Input: part model. Units: mm. Frame: model coordinates. A direction names the side the tool comes from. Give positions to 0.01 mm unless a question says otherwise; leave off trailing zeros. Order: outer loops, then holes, each group sorted by start corner. A loop starts at its lowest first (then second) coordinate and runs counter-clockwise, first axis right, second up. Notation, with made-up numbers: (-11, -15.75) - (30, -15.75) arc R14 ccw to (30, 1.25) - close; hole circle Ø10 at (69.25, 21.5). An arc over 180 degrees is marked (long way). Use a Markdown table: item, result.
Autodesk Inventor part; units mm, degrees
ref_plane "YZ Plane" through (0, 0, 0) normal (1, 0, 0) x (0, 1, 0)
ref_plane "XZ Plane" through (0, 0, 0) normal (0, 1, 0) x (-1, 0, 0)
ref_plane "XY Plane" through (0, 0, 0) normal (0, 0, 1) x (1, 0, 0)
sketch "Sketch1" plane through (0, 0, 0) normal (0, 0, 1) x (1, 0, 0)
  line L0 (-46.8353, 30.48) -> (46.8353, 30.48)
  arc A0 (0, 55.88) -> (-46.8353, 30.48) centre (0, 0) ccw
  arc A1 (46.8353, 30.48) -> (0, 55.88) centre (0, 0) ccw
extrude "Extrusion1" add sketch "Sketch1" against normal blind 12.7
sketch "Sketch2" plane through (0, 0, 0) normal (0, 0, 1) x (1, 0, 0)
  line L0 (-46.8353, 30.48) -> (46.8353, 30.48)
  arc A0 (46.8353, 30.48) -> (-46.8353, 30.48) centre (0, 0) ccw
  line L1 (0, 55.88) -> (0, 0)
  line L2 (0, 0) -> (46.8353, 30.48)
  line L3 (-46.8353, 30.48) -> (0, 0)
  line L4 (0, 0) -> (-26.6416, 49.1203)
  line L5 (0, 0) -> (26.6416, 49.1203)
  line L6 (-16.5866, 48.9387) -> (-20.0564, 52.6491)
  line L7 (-20.0564, 52.6491) -> (-18.578, 57.5092)
  line L8 (-18.578, 57.5092) -> (-13.6298, 58.659)
  line L9 (-13.6298, 58.659) -> (-10.16, 54.9486)
  line L10 (-10.16, 54.9486) -> (-11.6384, 50.0885)
  line L11 (-11.6384, 50.0885) -> (-16.5866, 48.9387)
  line L12 (16.5866, 48.9387) -> (11.6384, 50.0885)
  line L13 (11.6384, 50.0885) -> (10.16, 54.9486)
  line L14 (10.16, 54.9486) -> (13.6298, 58.659)
  line L15 (13.6298, 58.659) -> (18.578, 57.5092)
  line L16 (18.578, 57.5092) -> (20.0564, 52.6491)
  line L17 (20.0564, 52.6491) -> (16.5866, 48.9387)
  line L18 (11.6384, 50.0885) -> (16.5866, 48.9387)
  line L19 (16.5866, 48.9387) -> (16.1555, 47.0836)
  line L20 (16.1555, 47.0836) -> (11.2073, 48.2333)
  line L21 (11.2073, 48.2333) -> (11.6384, 50.0885)
  line L22 (-16.5866, 48.9387) -> (-11.6384, 50.0885)
  line L23 (-11.6384, 50.0885) -> (-11.2072, 48.2329)
  line L24 (-11.2072, 48.2329) -> (-16.1554, 47.0832)
  line L25 (-16.1554, 47.0832) -> (-16.5866, 48.9387)
  line L26 (-17.0874, 49.4743) -> (-11.425, 50.79)
  line L27 (11.425, 50.79) -> (17.0874, 49.4743)
  point P0 (-15.1082, 53.7989)
  point P1 (15.1082, 53.7989)
  dimension "d8" = 28.47
  dimension "d9" = 28.47
  dimension "d18" = 5.08
  dimension "d19" = 5.08
  dimension "d20" = 10.16
  dimension "d21" = 10.16
  dimension "d22" = 1.905
  dimension "d23" = 1.9046
  dimension "d24" = 0.635
  dimension "d25" = 0.635
extrude "Extrusion2" cut sketch "Sketch2" against normal blind 12.7 contours A0 L4 L0 | L0 L4 L3 | L5 L0 L2 | L6 L7 L8 L9 A0 | A0 L10 L26 L6 | L0 L5 A0 | L14 L15 L16 L17 A0 | A0 L17 L27 L13 | L11 L23 L24 L25 | L12 L19 L20 L21
sketch "Sketch3" plane through (-17.0874, 49.4743, 0) normal (-0.2263272, 0.9740513, 0) x (0.9740513, 0.2263272, 0)
  line L0 (0, 0) -> (0, 12.7)
  line L1 (1.0016, 8.763) -> (1.0016, 4.4937)
  line L2 (1.0016, 4.4937) -> (4.8116, 4.4937)
  line L3 (4.8116, 4.4937) -> (4.8116, 8.763)
  line L4 (4.8116, 8.763) -> (1.0016, 8.763)
  point P0 (5.8132, 12.7)
  point P1 (5.4466, 0)
  dimension "d28" = 0.635
  dimension "d29" = 3.81
  dimension "d30" = 3.937
extrude "Extrusion3" cut sketch "Sketch3" against normal up to next
sketch "Sketch4" plane through (11.425, 50.79, 0) normal (0.2263272, 0.9740513, 0) x (0.9740513, -0.2263272, 0)
  line L0 (0, 0) -> (0, 12.7)
  line L1 (0.635, 8.763) -> (0.635, 4.4958)
  line L2 (0.635, 4.4958) -> (4.445, 4.4958)
  line L3 (4.445, 4.4958) -> (4.445, 8.763)
  line L4 (4.445, 8.763) -> (0.635, 8.763)
  point P0 (0.3666, 0)
  dimension "d33" = 3.81
  dimension "d34" = 3.937
  dimension "d35" = 0.635
  dimension "d36" = 4.2672
extrude "Extrusion4" cut sketch "Sketch4" against normal up to next
sketch "Sketch5" plane through (0, 0, -12.7) normal (0, 0, -1) x (-1, 0, 0)
  line L0 (16.5316, 30.48) -> (-16.5316, 30.48)
  line L1 (-16.5316, 30.48) -> (16.5316, 30.48)
  line L2 (16.5316, 30.48) -> (16.5316, 33.655)
  line L3 (16.5316, 33.655) -> (-16.5316, 33.655)
  line L4 (-16.5316, 33.655) -> (-16.5316, 30.48)
  dimension "d39" = 3.175
extrude "Extrusion5" add sketch "Sketch5" along normal blind 9.525
sketch "Sketch7" plane through (-16.5316, 33.655, -12.7) normal (0, 1, 0) x (1, 0, 0)
  line L0 (33.0631, 9.525) -> (0, 9.525)
  line L1 (0, 9.525) -> (33.0631, 9.525)
  line L2 (33.0631, 9.525) -> (33.0631, 6.35)
  line L3 (33.0631, 6.35) -> (0, 6.35)
  line L4 (0, 6.35) -> (0, 9.525)
  point P0 (16.5316, -12.7)
  dimension "d42" = 3.175
extrude "Extrusion6" add sketch "Sketch7" along normal blind 6.35
sketch "Sketch8" plane through (0, 0, 0) normal (0, 0, 1) x (1, 0, 0)
  line L0 (-16.5316, 30.48) -> (16.5316, 30.48)
  line L1 (-16.5316, 30.48) -> (16.5316, 30.48)
  line L2 (16.5316, 30.48) -> (16.5316, 33.655)
  line L3 (16.5316, 33.655) -> (-16.5316, 33.655)
  line L4 (-16.5316, 33.655) -> (-16.5316, 30.48)
  dimension "d45" = 3.175
extrude "Extrusion7" add sketch "Sketch8" along normal blind 9.525
sketch "Sketch9" plane through (-16.5316, 33.655, 0) normal (0, 1, 0) x (1, 0, 0)
  line L0 (0, -9.525) -> (33.0631, -9.525)
  line L1 (0, -9.525) -> (33.0631, -9.525)
  line L2 (33.0631, -9.525) -> (33.0631, -6.35)
  line L3 (33.0631, -6.35) -> (0, -6.35)
  line L4 (0, -6.35) -> (0, -9.525)
  point P0 (16.5316, 0)
  dimension "d48" = 3.175
extrude "Extrusion8" add sketch "Sketch9" along normal blind 6.35
properties part number "IR Sensor Piece Ver 2"
1. Mould query, pull axis X, two halves, no side actions, for faces 6 (the face through (11.42, 49.15, -6.26)), 7 (the face through (-23.185, 50.843, -6.261)), 8 (the face through (16.374, 48.024, -6.261)), 9 (the face through (23.28, 50.8, -6.26)). Classes: pulls with the +X half, pulls with the -X half, needs draft (parallel to the pull), parting line crosses it, or undercut.
Response:
| item | result |
|---|---|
| face 6 | undercut |
| face 7 | pulls with the -X half |
| face 8 | undercut |
| face 9 | pulls with the +X half |
2. Material intervals for line 1 along Z through (x, y) = (-6, 36.25) (3 decimals); line 2 along Z through (x, y) = (-15.5, 40.25); line 3 along Y through (x, z) = (13.5, -20) (3 decimals), sorted ascending.
Response:
| item | result |
|---|---|
| line 1 | z = -22.225 to -19.05, -12.7 to 0, 6.35 to 9.525 |
| line 2 | z = -12.7 to 0 |
| line 3 | y = 30.48 to 40.005 |
3. Section query A-A (y = 38.75). State how many separate pieces and enclosed holes the cut face has, then the cut area to 3 significant figures.
Response:
| item | result |
|---|---|
| separate pieces | 3 |
| enclosed holes | 0 |
| area | 744 mm^2 |
4. Pin query (flat end, axial travel): pin 1 (3 mm diameter, centred on x = -7, z = 4.5, fed in from +Y) (3 decimals); pin 2 (3 mm diameter, centred on x = 9.5, z = -10.5, fed in from +Y); pin 3 (0.7 mm diameter, centred on x = 14, y = 49.5, fed in from +Z). Return the tip coordinate at first contact, or that it passes through.
Response:
| item | result |
|---|---|
| pin 1 | stops at y = 33.655 |
| pin 2 | stops at y = 55.3 |
| pin 3 | stops at z = 0 |
5. Section query B-B (x = -4). Return loops of the section in (y, z) (3 decimals).
Response:
| item | result |
|---|---|
| outline | (30.48, -22.225) - (40.005, -22.225) - (40.005, -19.05) - (33.655, -19.05) - (33.655, -12.7) - (55.737, -12.7) - (55.737, 0) - (33.655, 0) - (33.655, 6.35) - (40.005, 6.35) - (40.005, 9.525) - (30.48, 9.525) - close |
6. Set-up query: faces 1 (the face through (0, 40.005, -21)), 2 (the face through (15.8, 49.12, -6.26)), 3 (the face through (16.104, 49.703, -6.261)), 4 (the face through (-16.532, 34, 7)), 5 (the face through (0, 33.655, 3)). Return all of +Z, -Z, +X, -X, +Y, -Y with unobstructed straight access to the full face (end or side cutting, diameter ignored); none if empty.
Response:
| item | result |
|---|---|
| face 1 | -Z, +X, -X, +Y |
| face 2 | +Z, -Z |
| face 3 | +Z, -Z, +Y |
| face 4 | +Z, -X, +Y, -Y |
| face 5 | +X, -X, +Y |
